from build123d import *

# Parameters (mm, degrees)
SKETCH1_R           = 20
SKETCH1_R_2         = 5
BOSS_EXTRUDE1_DEPTH = 2
BOSS_EXTRUDE2_DEPTH = 30
FILLET1_R           = 2.5


with BuildPart() as part:
    # Sketch1 → Boss-Extrude1 (new body)
    with BuildSketch(Plane.XY):
        Circle(SKETCH1_R)
        Circle(SKETCH1_R_2, mode=Mode.SUBTRACT)
    extrude(amount=BOSS_EXTRUDE1_DEPTH)

    # Sketch2 → Boss-Extrude2 (add)
    with BuildSketch(Plane.XY.offset(2)):
        with BuildLine():
            Line((-2.625, -19.826986029), (-2.625, -17.2514311))
            ThreePointArc((-2.625, -17.2514311), (-11.373131715, 13.234590096), (17.45, 0))
            ThreePointArc((17.45, 0), (13.234590096, -11.373131715), (2.625, -17.2514311))
            Line((2.625, -17.2514311), (2.625, -19.826986029))
            ThreePointArc((2.625, -19.826986029), (15.041608956, -13.181426326), (20, 0))
            ThreePointArc((20, 0), (-13.181426326, 15.041608956), (-2.625, -19.826986029))
        make_face()
    extrude(amount=BOSS_EXTRUDE2_DEPTH)

    # Fillet1
    fillet1_edges = [part.edges().sort_by_distance(p)[0] for p in [
        (-2.625, -17.2514311, 17),
        (2.625, -17.2514311, 17),
    ]]
    fillet(fillet1_edges, radius=FILLET1_R)


solid = part.part
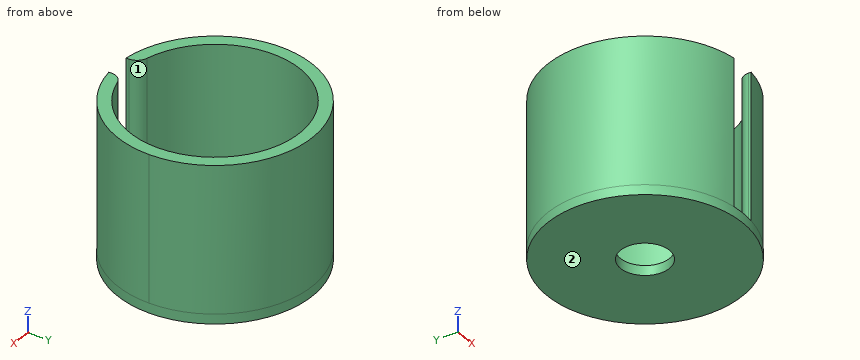
The listing builds one solid part. Answer for the finished solid, in the listing's coordinates (mm). Face numbers are marked on the shaded views. Coordinates: 2 decimals unless noted, no trailing zeros. Write each loop counter-clockwise with the first axis right and the second up, starting at its lowest first coordinate (ties: lowest second). Pieces come first, ordered by that corner, then holes. Notation, with made-up numbers: (35.25, 87) - (72.25, 87) arc R25 ccw to (72.25, 106) - close; hole circle Ø3 at (-17.75, -28.75). An arc over 180 degrees is marked (long way). Put each result on its own line as item: value.
1. Flat-ended cylindrical pins translate along their axes: pin 1 Ø2 at (y, z) = (-7.5, 27.5) entering from -X; pin 2 Ø8 at (x, z) = (-7.5, 5.5) entering from -Y; pin 3 Ø12 at (y, z) = (-11, 8.5) entering from -X. Find the tip coordinate at first contact, or state that the pin passes through.
Answer sheet:
pin 1: stops at x = -18.91
pin 2: stops at y = -19.69
pin 3: stops at x = -19.36
2. Determine the mould class of the marked faces 1 and 2 for opening direction X: pulls with the +X half, pulls with the -X half, needs draft (parallel to the pull), parting line crosses it, or undercut.
Answer sheet:
face 1: undercut
face 2: needs draft
3. The part is cut by section B-B on y = 4. Give the vertices of the cut face in (x, z).
Answer sheet:
outline: (-19.6, 0) - (-3, 0) - (-3, 2) - (-16.99, 2) - (-16.99, 32) - (-19.6, 32) - close; (3, 0) - (19.6, 0) - (19.6, 32) - (16.99, 32) - (16.99, 2) - (3, 2) - close
4. The part is cut by section A-A on x = 0. Give the vertices of the cut face in (y, z).
Answer sheet:
outline: (-20, 0) - (-5, 0) - (-5, 2) - (-20, 2) - close; (5, 0) - (20, 0) - (20, 32) - (17.45, 32) - (17.45, 2) - (5, 2) - close
5. The part is cut by section D-D on x = 9. Give the vertices of the cut face in (y, z).
Answer sheet:
outline: (-17.86, 0) - (17.86, 0) - (17.86, 32) - (14.95, 32) - (14.95, 2) - (-14.95, 2) - (-14.95, 32) - (-17.86, 32) - close
6. The part is cut by section C-C on z = 11. Give the vertices of the cut face in (x, y) (3 decimals), plus the area to 3 significant figures.
Answer sheet:
outline: (-4.483, -16.864) arc R17.45 cw (long way) to (4.483, -16.864) arc R2.5 ccw to (2.625, -19.28) - (2.625, -19.827) arc R20 ccw (long way) to (-2.625, -19.827) - (-2.625, -19.28) arc R2.5 ccw to start
area: 285 mm^2
7. Find the intervals of material crossed by line 1 along X through (y, z) = (0.5, 14.5); line 2 along Y through (x, z) = (0, 0.7); line 3 along Z through (x, y) = (10, -6), in increasing order. Write a range as from..to.
Answer sheet:
line 1: x = -19.99..-17.44, 17.44..19.99
line 2: y = -20..-5, 5..20
line 3: z = 0..2
